from build123d import *

# Parameters (mm, degrees)
BOSS_EXTRUDE1_DEPTH = 5.08
SKETCH3_R           = 11.00455
SKETCH3_R_2         = 3.175
CUT_EXTRUDE2_DEPTH  = 5.08
SKETCH4_W           = 38.1
SKETCH4_H           = 3.81
CUT_EXTRUDE3_DEPTH  = 6.08


with BuildPart() as part:
    # Sketch1 → Boss-Extrude1 (new body)
    with BuildSketch(Plane.XY):
        Polygon((-44.45, 38.1), (44.45, 38.1), (12.7, 0), (-12.7, 0), align=None)
    extrude(amount=BOSS_EXTRUDE1_DEPTH)

    # Sketch3 → Cut-Extrude2 (cut)
    with BuildSketch(Plane.XY.offset(5.08)):
        with Locations((0, 19.05)):
            Circle(SKETCH3_R)
        with Locations((-25.4, 31.75)):
            Circle(SKETCH3_R_2)
        with Locations((25.4, 31.75)):
            Circle(SKETCH3_R_2)
        Polygon((-33.02, 24.384), (-33.02, 38.1), (-44.45, 38.1), align=None)
        Polygon((33.02, 38.1), (33.02, 24.384), (44.45, 38.1), align=None)
    extrude(amount=-CUT_EXTRUDE2_DEPTH, mode=Mode.SUBTRACT)

    # Sketch4 → Cut-Extrude3 (cut, through all)
    with BuildSketch(Plane.XY.offset(5.08)):
        with Locations((0, 1.905)):
            Rectangle(SKETCH4_W, SKETCH4_H)
    extrude(amount=-CUT_EXTRUDE3_DEPTH, mode=Mode.SUBTRACT)


solid = part.part
Build history of the part. All positions in model axes, mm. Coordinates: 2 decimals unless noted, no trailing zeros. Order: outer loops, then holes, each group sorted by start corner. A loop starts at its lowest first (then second) coordinate and runs counter-clockwise, first axis right, second up. Notation, with made-up numbers: (-27.75, 35.25) -> (0.25, 35.25) arc R6 cw to (0.25, 45.25) -> close; hole circle Ø3 at (-7.5, 38.5). An arc over 180 degrees is marked (long way). One line per item, written item: value.
(1) Slice it at B-B, the plane y = 19.05. List the corners of the cut face in (x, z) (3 decimals).
Checked values:
outline: (-28.575, 0) -> (-11.005, 0) -> (-11.005, 5.08) -> (-28.575, 5.08) -> close; (11.005, 0) -> (28.575, 0) -> (28.575, 5.08) -> (11.005, 5.08) -> close
(2) Slice it at D-D, the plane y = 31.75. List the corners of the cut face in (x, z) (3 decimals), plus the area to 3 significant figures.
Checked values:
outline: (-33.02, 0) -> (-28.575, 0) -> (-28.575, 5.08) -> (-33.02, 5.08) -> close; (-22.225, 0) -> (22.225, 0) -> (22.225, 5.08) -> (-22.225, 5.08) -> close; (28.575, 0) -> (33.02, 0) -> (33.02, 5.08) -> (28.575, 5.08) -> close
area: 271 mm2
(3) Probe line 1 (X direction, y = 31.5, z = 1.05); line 2 (Y direction, x = 0, z = 1.2); line 3 (Y direction, x = -25.4, z = 3.45) (3 decimals). List the from-to ranges inside material, lowest first. Write a range as [from, to].
Checked values:
line 1: [-33.02, -28.57], [-22.23, 22.23], [28.57, 33.02]
line 2: [3.81, 8.05], [30.05, 38.1]
line 3: [15.24, 28.575], [34.925, 38.1]
(4) Drop flat-ended pins along their axis: pin 1 Ø7.5 at (x, y) = (-25.4, 31.75) entering from +Z; pin 2 Ø17.5 at (x, y) = (0, 19.05) entering from +Z. Give the stop position or say it passes through.
Checked values:
pin 1: z = 5.08
pin 2: through
(5) Mould opens along Y. For faces 1 (the cylindrical face through (-8.1, 26.5, 2.6)), 2 (the flat face through (0, 38.1, 3)), 3 (the flat face through (24.568, 14.241, 2.504)) say: pulls with the +Y half, pulls with the -Y half, needs draft (parallel to the pull), parting line crosses it, or undercut.
Checked values:
face 1: undercut
face 2: pulls with the +Y half
face 3: pulls with the -Y half
(6) Slice it at C-C, the plane z = 3.2. List the corners of the cut face in (x, y) (3 decimals).
Checked values:
outline: (-33.02, 24.384) -> (-15.875, 3.81) -> (15.875, 3.81) -> (33.02, 24.384) -> (33.02, 38.1) -> (-33.02, 38.1) -> close; hole circle Ø6.35 at (-25.4, 31.75); hole circle Ø22.009 at (0, 19.05); hole circle Ø6.35 at (25.4, 31.75)
(7) Slice it at A-A, the plane x = 25.4. List the corners of the cut face in (y, z) (3 decimals).
Checked values:
outline: (15.24, 0) -> (28.575, 0) -> (28.575, 5.08) -> (15.24, 5.08) -> close; (34.925, 0) -> (38.1, 0) -> (38.1, 5.08) -> (34.925, 5.08) -> close
